```python
from build123d import *

# Parameters (mm, degrees)
PAD017_DEPTH = 20
PAD015_DEPTH = 33
PAD016_DEPTH = 20
FILLET010_R  = 1
FILLET011_R  = 0.4
FILLET012_R  = 1.5
FILLET013_R  = 2


with BuildPart() as pad017:
    # Sketch021 → Pad017 (new body)
    with BuildSketch(Plane(origin=(10, -7, 0.4), x_dir=(1, 0, 0), z_dir=(0, -1, 0))):
        Polygon((12.921668, -76.043343), (12.921668, -72.681298), (10.907037, -71.064545), (12.949577, -67.987406), (17.894252, -67.987406), (19.953335, -71.012405), (17.993304, -72.648705), (17.981073, -76.043343), align=None)
    extrude(amount=PAD017_DEPTH)


with BuildPart() as pad015:
    # Sketch019 → Pad015 (new body)
    with BuildSketch(Plane.XZ):
        Polygon((31.922119, -73.764191), (34.715668, -84.347412), (31.00419, -84.347412), (29.994871, -83.010223), (29.004835, -82.997353), (29.97435, -84.356453), (27.001257, -84.356453), (25.99424, -83.013763), (24.977634, -83.013763), (26.003832, -84.375633), (23.007538, -84.375633), (22.019703, -83.023636), (20.974325, -83.023636), (22.000523, -84.366325), (19.017838, -84.366325), (17.99164, -83.004456), (16.984625, -83.004456), (18.00123, -84.366325), (15.032244, -84.366325), (14.013124, -83.020378), (12.982291, -83.020378), (14.00141, -84.379204), (12.681671, -84.379204), (4.650895, -73.764191), align=None)
    extrude(amount=PAD015_DEPTH)


with BuildPart() as fillet013:
    # Sketch020 → Pad016 (new body)
    with BuildSketch(Plane(origin=(-4, -7, 0.4), x_dir=(1, 0, 0), z_dir=(0, -1, 0))):
        Polygon((12.921668, -76.043343), (12.921668, -72.681298), (10.907037, -71.064545), (12.949577, -67.987406), (17.894252, -67.987406), (19.953335, -71.012405), (17.993304, -72.648705), (17.981073, -76.043343), align=None)
    extrude(amount=PAD016_DEPTH)

    # Fusion002: union Pad015
    add(pad015.part)

    # Fusion003: union Pad017
    add(pad017.part)

    # Fillet010
    fillet010_edges = [fillet013.edges().sort_by_distance(p)[0] for p in [
        (20.907037, -17, -70.664545),
        (22.949577, -17, -67.587406),
        (27.894252, -17, -67.587406),
        (29.953335, -17, -70.612405),
        (15.953335, -17, -70.612405),
        (13.894252, -17, -67.587406),
        (8.949577, -17, -67.587406),
        (6.907037, -17, -70.664545),
    ]]
    fillet(fillet010_edges, radius=FILLET010_R)

    # Fillet011
    fillet011_edges = [fillet013.edges().sort_by_distance(p)[0] for p in [
        (22.921668, -17, -73.764191),
        (27.987844, -17, -73.764191),
        (8.921668, -17, -73.764191),
        (13.987844, -17, -73.764191),
    ]]
    fillet(fillet011_edges, radius=FILLET011_R)

    # Fillet012
    fillet012_edges = [fillet013.edges().sort_by_distance(p)[0] for p in [
        (12.681671, -16.5, -84.379204),
    ]]
    fillet(fillet012_edges, radius=FILLET012_R)

    # Fillet013
    fillet013_edges = [fillet013.edges().sort_by_distance(p)[0] for p in [
        (34.715668, -16.5, -84.347412),
    ]]
    fillet(fillet013_edges, radius=FILLET013_R)


solid = fillet013.part
```
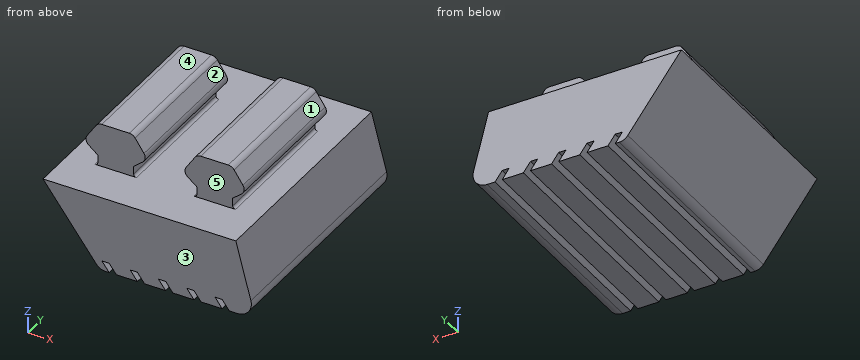
Check sheet for the modelled part. Datum: model origin and axes. Units: mm. Face numbers are marked on the shaded views. A direction names the side the tool comes from. Coordinates: 2 decimals unless noted, no trailing zeros. Write each loop counter-clockwise with the first axis right and the second up, starting at its lowest first coordinate (ties: lowest second). Pieces come first, ordered by that corner, then holes. Notation, with made-up numbers: M 59.25,-16 L 102.25,-16 A15 ccw 102.25,-7 Z; hole C 49.25,1.25 d2. An arc over 180 degrees is marked long. Use one line per item in the form item = value.
Item 1: Material ranges on L1, parallel to X at y = -17.5, z = -72; L2, parallel to Z at x = 28.5, y = -23.5; L3, parallel to X at y = -20.5, z = -69, recorded low to high. Write a range as from..to.
Answer below:
L1 = 8.57..14.29, 22.57..28.29
L2 = -84.36..-73.76, -71.83..-68.48
L3 = 8.01..14.86, 22.01..28.86
Item 2: Gauge pin test, flat ends, axial feed: pin 1 Ø5 at (y, z) = (-10, -70) entering from +X; pin 2 Ø3 at (x, z) = (11, -70) entering from -Y; pin 3 Ø1.9 at (x, z) = (25, -71) entering from +Y; pin 4 Ø8 at (y, z) = (-12.5, -79) entering from +X. Record the tip position at first contact, or that the pin passes through.
Answer below:
pin_1 = 29.62
pin_2 = -27
pin_3 = -7
pin_4 = 34.12
Item 3: Sectioned sample at C-C, the plane x = 11.5. Record the cut outline in (y, z).
Answer below:
outline = M -33,-82.82 L 0,-82.82 L 0,-73.76 L -7,-73.76 L -7,-67.59 L -27,-67.59 L -27,-73.76 L -33,-73.76 Z
Item 4: Sectioned sample at D-D, the plane z = -79.5. Record the cut outline in (x, y), and give its area (3 significant figures).
Answer below:
outline = M 8.99,-33 L 33.44,-33 L 33.44,0 L 8.99,0 Z
area = 807 mm^2
Item 5: Set-up check for the marked faces 4 and 5: record each of +Z, -Z, +X, -X, +Y, -Y from which the full face is reachable in a straight line by a thin tool's end or side.
Answer below:
face_4 = +Z, +X, -X, +Y, -Y
face_5 = +Z, +X, -X, -Y
Item 6: Release check for a two-part mould opening along X. For the marked faces 1, 2 and 3 record: pulls with the +X half, pulls with the -X half, needs draft (parallel to the pull), parting line crosses it, or undercut.
Answer below:
face_1 = pulls with the +X half
face_2 = undercut
face_3 = needs draft
Item 7: Sectioned sample at A-A, the plane x = 24. Record the cut outline in (y, z).
Answer below:
outline = M -33,-84.38 L 0,-84.38 L 0,-73.76 L -7,-73.76 L -7,-67.59 L -27,-67.59 L -27,-73.76 L -33,-73.76 Z
Item 8: Sectioned sample at B-B, the plane z = -82.25. Record the cut outline in (x, y), and give its area (3 significant figures).
Answer below:
outline = M 11.07,-33 L 34.12,-33 L 34.12,0 L 11.07,0 Z
area = 761 mm^2
